Input: part model. Units: mm. Frame: model coordinates. A direction names the side the tool comes from. Round coordinates to 2 decimals unless told otherwise and drop trailing zeros. Order: outer loops, then holes, each group sorted by start corner. A loop starts at its lowest first (then second) coordinate and runs counter-clockwise, first axis right, second up.
Item 1: Reachability of faces 1 (the cylindrical face through (42.994, 20.591, 5.635)), 2 (the flat face through (25, 18, 11.43)) from +Z, -Z, +X, -X, +Y, -Y: full face, straight path, thin tool, end or side. Return the list, or none.
Item 2: Cut plane B-B on x = 38.1. Output: boundary loops of the cut face in (y, z), then the cut area to 3 significant figures.
Item 3: Cut plane C-C on z = 19.05. Output: boundary loops of the cut face in (x, y), then the cut area to 3 significant figures.
Item 4: Mould query, pull axis Z, two halves, no side actions, for faces 3 (the cylindrical face through (28.89, 4.44, 17.59)), 4 (the flat face through (25, 13, 0)), 5 (the flat face through (25, 5, 25.4)), 6 (the cylindrical face through (11.66, 14.35, 5.63)). Classes: released by +Z, released by -Z, zero draft, split by the parting line, or undercut.
Item 5: Cut plane D-D on z = 5.5. Output: boundary loops of the cut face in (x, y).
Item 6: Line query: L1, parallel to X at y = 4.5, z = 19.05; L2, parallel to X at y = 17.75, z = 9.75; L3, parallel to Y at x = 12.7, z = 6.5. Output: solid intervals per line, ascending.
Item 7: Cut plane A-A on y = 19.05. Output: boundary loops of the cut face in (x, z), then the cut area to 3 significant figures.
Item 8: First-contact query: pin 1 (3 mm diameter, centred on x = 9, y = 21.5, fed in from -Z); pin 2 (11 mm diameter, centred on x = 28, z = 17.5, fed in from +Y); pin 3 (4.5 mm diameter, centred on x = 14, y = 16.5, fed in from +Z). Flat tips, straight axial feed; report the tip coordinate or a pass-through.
```python
from build123d import *

# Parameters (mm, degrees)
SKETCH1_W                                         = 50.8
SKETCH1_H                                         = 25.4
SKETCH1_R                                         = 4.8133
SKETCH1_R_2                                       = 5.1308
BOSS_EXTRUDE1_DEPTH                               = 11.43
SKETCH2_W                                         = 50.8
SKETCH2_H                                         = 25.4
BOSS_EXTRUDE2_DEPTH                               = 10.16
CSK_FOR_4_FLAT_HEAD_MACHINE_SCREW_100_D           = 2.9464
CSK_FOR_4_FLAT_HEAD_MACHINE_SCREW_100_CSINK_D     = 5.715
CSK_FOR_4_FLAT_HEAD_MACHINE_SCREW_100_CSINK_ANGLE = 100


with BuildPart() as part:
    # Sketch1 → Boss-Extrude1 (new body)
    with BuildSketch(Plane.XY):
        with Locations((25.4, 12.7)):
            Rectangle(SKETCH1_W, SKETCH1_H)
        with Locations((12.7, 19.05)):
            Circle(SKETCH1_R, mode=Mode.SUBTRACT)
        with Locations((38.1, 19.05)):
            Circle(SKETCH1_R_2, mode=Mode.SUBTRACT)
    extrude(amount=BOSS_EXTRUDE1_DEPTH)

    # Sketch2 → Boss-Extrude2 (add)
    with BuildSketch(Plane(origin=(0, 0, 0), x_dir=(1, 0, 0), z_dir=(0, 1, 0))):
        with Locations((25.4, -12.7)):
            Rectangle(SKETCH2_W, SKETCH2_H)
    extrude(amount=BOSS_EXTRUDE2_DEPTH)

    # CSK for #4 Flat Head Machine Screw (100)1 (through all)
    with Locations(Plane(origin=(0, 10.16, 0), x_dir=(1, 0, 0), z_dir=(0, 1, 0))):
        with Locations((28.702, -19.05), (6.35, -19.05)):
            CounterSinkHole(CSK_FOR_4_FLAT_HEAD_MACHINE_SCREW_100_D / 2, CSK_FOR_4_FLAT_HEAD_MACHINE_SCREW_100_CSINK_D / 2, counter_sink_angle=CSK_FOR_4_FLAT_HEAD_MACHINE_SCREW_100_CSINK_ANGLE)


solid = part.part
```
From the geometry:
1. face 1: +Z, -Z
1. face 2: +Z, +X, -X, +Y
2. outline: (0, 0) - (13.92, 0) - (13.92, 11.43) - (10.16, 11.43) - (10.16, 25.4) - (0, 25.4) - close; (24.18, 0) - (25.4, 0) - (25.4, 11.43) - (24.18, 11.43) - close
2. area: 315 mm2
3. outline: (0, 0) - (4.88, 0) - (4.88, 9) - (3.49, 10.16) - (0, 10.16) - close; (7.82, 0) - (27.23, 0) - (27.23, 9) - (25.84, 10.16) - (9.21, 10.16) - (7.82, 9) - close; (30.18, 0) - (50.8, 0) - (50.8, 10.16) - (31.56, 10.16) - (30.18, 9) - close
3. area: 453 mm2
4. face 3: undercut
4. face 4: released by -Z
4. face 5: released by +Z
4. face 6: zero draft
5. outline: (0, 0) - (50.8, 0) - (50.8, 25.4) - (0, 25.4) - close; hole circle Ø9.63 at (12.7, 19.05); hole circle Ø10.26 at (38.1, 19.05)
6. L1: x = 0 to 4.88, 7.82 to 27.23, 30.18 to 50.8
6. L2: x = 0 to 8.07, 17.33 to 33.14, 43.06 to 50.8
6. L3: y = 0 to 14.24, 23.86 to 25.4
7. outline: (0, 0) - (7.89, 0) - (7.89, 11.43) - (0, 11.43) - close; (17.51, 0) - (32.97, 0) - (32.97, 11.43) - (17.51, 11.43) - close; (43.23, 0) - (50.8, 0) - (50.8, 11.43) - (43.23, 11.43) - close
7. area: 353 mm2
8. pin 1: stops at z = 0
8. pin 2: stops at y = 10.16
8. pin 3: stops at z = 11.43
